Could you check a few things on this model? Use its own coordinates, in mm. Round coordinates to 2 decimals unless told otherwise and drop trailing zeros. Order: outer loops, then holes, each group sorted by start corner. A loop starts at its lowest first (then second) coordinate and runs counter-clockwise, first axis right, second up. Notation, with made-up numbers: (-31.5, 16.25) - (10.5, 16.25) arc R9 ccw to (10.5, 30.25) - close; hole circle Ø10 at (63, 13). An arc over 180 degrees is marked (long way). Use one line per item in the form item = value.
from build123d import *

# Parameters (mm, degrees)
EXTRUDE_1_DEPTH     = 3
SKETCH_2_R          = 1.6
CUT_EXTRUDE_1_DEPTH = 56.253959134


with BuildPart() as part:
    # 草图1 → 凸台-拉伸1 (new body)
    with BuildSketch(Plane.XY):
        Polygon((0, 0), (20, 0), (40, -23), (40, -38), (-20, -38), (-20, -23), align=None)
    extrude(amount=EXTRUDE_1_DEPTH)

    # 草图2 → 切除-拉伸1 (cut, through all)
    with BuildSketch(Plane.XY.offset(3)):
        with Locations((-15, -34.25)):
            Circle(SKETCH_2_R)
        with Locations(Location((-15, -26.75, 0), (0, 0, 180))):
            Circle(SKETCH_2_R)
        with Locations(Location((-5, -34.25, 0), (0, 0, 180))):
            Circle(SKETCH_2_R)
        with Locations((-5, -26.75)):
            Circle(SKETCH_2_R)
        with Locations((25, -34.25)):
            Circle(SKETCH_2_R)
        with Locations(Location((35, -34.25, 0), (0, 0, 180))):
            Circle(SKETCH_2_R)
        with Locations(Location((25, -26.75, 0), (0, 0, 180))):
            Circle(SKETCH_2_R)
        with Locations((35, -26.75)):
            Circle(SKETCH_2_R)
        with Locations((5, -5)):
            Circle(SKETCH_2_R)
        with Locations(Location((15, -5, 0), (0, 0, 180))):
            Circle(SKETCH_2_R)
        with Locations((15, -15)):
            Circle(SKETCH_2_R)
        with Locations(Location((5, -15, 0), (0, 0, 180))):
            Circle(SKETCH_2_R)
    extrude(amount=-CUT_EXTRUDE_1_DEPTH, mode=Mode.SUBTRACT)


solid = part.part
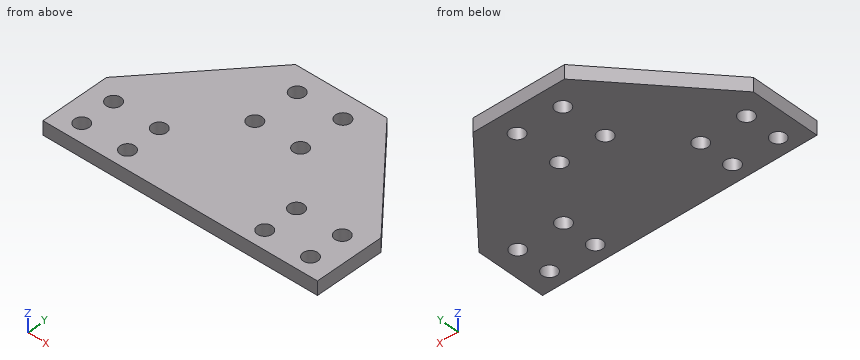
Item 1: Imagine slicing it at C-C on z = 1.2. State how many separate pieces and enclosed holes the cut face has, plus the area to 3 significant figures.
Found:
separate_pieces = 1
enclosed_holes = 12
area = 1,720 mm2
Item 2: Imagine slicing it at D-D on y = -15. Please give me the cut outline in (x, z), plus the area to 3 significant figures.
Found:
outline = (-13.04, 0) - (3.4, 0) - (3.4, 3) - (-13.04, 3) - close; (6.6, 0) - (13.4, 0) - (13.4, 3) - (6.6, 3) - close; (16.6, 0) - (33.04, 0) - (33.04, 3) - (16.6, 3) - close
area = 119 mm2
Item 3: Will these pins go through, and if not, where does the flat tip stop? P1, Ø1, axis at y = -17.5, z = 0.5, coming from the +X side; P2, Ø3, axis at x = -15, y = -26.75, coming from the +Z side.
Found:
P1 = 35.65
P2 = through
Item 4: Imagine slicing it at A-A on x = 15. Please give me the cut outline in (y, z).
Found:
outline = (-38, 0) - (-16.6, 0) - (-16.6, 3) - (-38, 3) - close; (-13.4, 0) - (-6.6, 0) - (-6.6, 3) - (-13.4, 3) - close; (-3.4, 0) - (0, 0) - (0, 3) - (-3.4, 3) - close
Item 5: I need wall thicknesses on L1, parallel to Y at x = -5, z = 2.2; L2, parallel to Y at x = 35, z = 1.3; L3, parallel to Y at x = 30.5, z = 0.6 (3 decimals). Which ranges of each line are inside material? Lowest first, please.
Found:
L1 = -38 to -35.85, -32.65 to -28.35, -25.15 to -5.75
L2 = -38 to -35.85, -32.65 to -28.35, -25.15 to -17.25
L3 = -38 to -12.075
Item 6: Imagine slicing it at B-B on y = -26.75. Please give me the cut outline in (x, z), plus the area to 3 significant figures.
Found:
outline = (-20, 0) - (-16.6, 0) - (-16.6, 3) - (-20, 3) - close; (-13.4, 0) - (-6.6, 0) - (-6.6, 3) - (-13.4, 3) - close; (-3.4, 0) - (23.4, 0) - (23.4, 3) - (-3.4, 3) - close; (26.6, 0) - (33.4, 0) - (33.4, 3) - (26.6, 3) - close; (36.6, 0) - (40, 0) - (40, 3) - (36.6, 3) - close
area = 142 mm2
